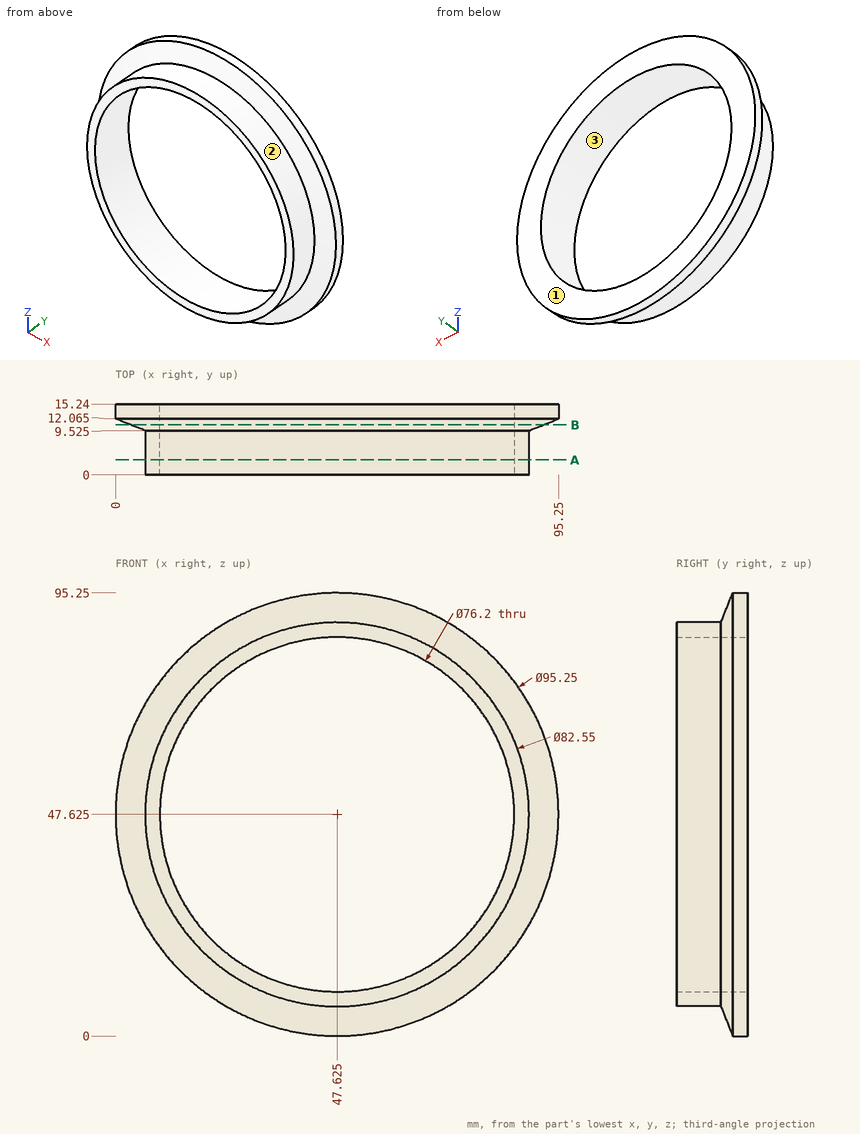
Study the drawing (mm; zero at the part's minimum x, y, z) and answer. Coordinates: 2 decimals unless noted, no trailing zeros. Order: outer loops, then holes, each group sorted by start corner. A loop starts at its lowest first (then second) coordinate and runs counter-clockwise, first axis right, second up. Notation, with made-up numbers: M 78.25,17.5 L 137.25,17.5 A26 ccw 137.25,39.5 Z; hole C 48,48 d1. An arc over 180 degrees is marked long. Answer as a JSON object with one key per item and string values. Group by question number.
1. Flat-ended cylindrical pins translate along their axes: P1, Ø4, axis at y = 12.5, z = 64.5, coming from the +X side; P2, Ø1.5, axis at x = 53, y = 13.5, coming from the -Z side; P3, Ø3, axis at x = 28.5, y = 1.5, coming from the -Z side. Find the tip coordinate at first contact, or state that the pin passes through.
2. Determine the mould class of the marked faces 1, 2 and 3 for opening direction Z: released by +Z, released by -Z, zero draft, split by the parting line, or undercut.
3. Section B-B on y = 10.75 is taken. Write down the section's boundary in (x, z) (1 decimal), then the cut area to 3 significant figures.
4. Straight lines are drawn through the part: line 1 (Z direction, x = 46.5, y = 13); line 2 (X direction, y = 8.5, z = 77); line 3 (Z direction, x = 26.5, y = 4.5). For each, find the intervals that lie inside material, in ascending order.
5. Section A-A on y = 3.25 is taken. Write down the section's boundary in (x, z) (3 decimals).
Values follow:
{
 "1": {"P1": "x = 92.87", "P2": "z = 0.23", "P3": "z = 10.3"},
 "2": {"face 1": "zero draft", "face 2": "split by the parting line", "face 3": "undercut"},
 "3": {"outline": "C 47.6,47.6 d88.7; hole C 47.6,47.6 d76.2", "area": "1,620 mm2"},
 "4": {"line 1": "0.01 to 9.54, 85.71 to 95.24", "line 2": "18.63 to 23.36, 71.89 to 76.62", "line 3": "12.17 to 15.92, 79.33 to 83.08"},
 "5": {"outline": "C 47.625,47.625 d82.55; hole C 47.625,47.625 d76.2"}
}
